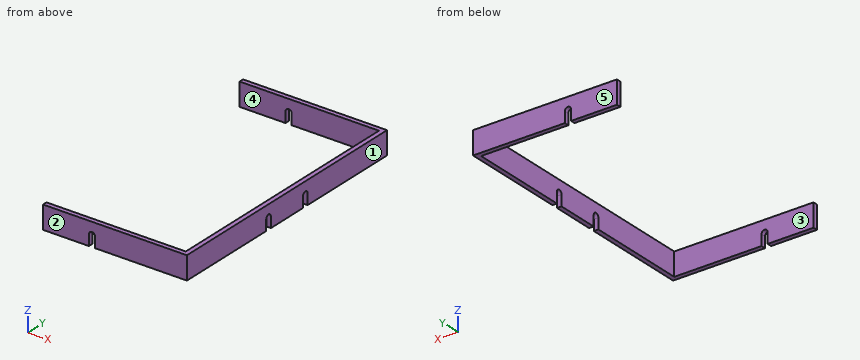
```python
from build123d import *

# Parameters (mm, degrees)
F0_W     = 94
F0_H     = 174
F1_DEPTH = 15
F2_T     = -3
F4_DEPTH = 100
F6_DEPTH = 125


with BuildPart() as f1:
    # F0 (on Top) → F1 (new body)
    with BuildSketch(Plane.XY):
        Rectangle(F0_W, F0_H)
    extrude(amount=F1_DEPTH)

    # F2
    f2_openings = [f1.faces().sort_by_distance(p)[0] for p in [
        (0, 0, 15),
        (-47, 0, 7.5),
        (0, 0, 0),
    ]]
    offset(amount=F2_T, openings=f2_openings)

    # F3 (on Right) → F4 (cut)
    with BuildSketch(Plane.YZ):
        with BuildLine():
            Line((-18, 7), (-14, 7))
            ThreePointArc((-14, 7), (-16, 9), (-18, 7))
        make_face()
        with BuildLine():
            Line((-14, 0), (-14, 7))
            ThreePointArc((-14, 7), (-16, 5), (-18, 7))
            Line((-18, 7), (-18, 0))
            Line((-18, 0), (-14, 0))
        make_face()
        with BuildLine():
            ThreePointArc((-18, 7), (-16, 5), (-14, 7))
            Line((-14, 7), (-18, 7))
        make_face()
        with BuildLine():
            Line((14, 7), (18, 7))
            ThreePointArc((18, 7), (16, 9), (14, 7))
        make_face()
        with BuildLine():
            Line((18, 0), (18, 7))
            ThreePointArc((18, 7), (16, 5), (14, 7))
            Line((14, 7), (14, 0))
            Line((14, 0), (18, 0))
        make_face()
        with BuildLine():
            ThreePointArc((14, 7), (16, 5), (18, 7))
            Line((18, 7), (14, 7))
        make_face()
    extrude(amount=F4_DEPTH, mode=Mode.SUBTRACT)

    # F5 (on Front) → F6 (cut, symmetric)
    with BuildSketch(Plane.XZ):
        with BuildLine():
            Line((-17, 7), (-13, 7))
            ThreePointArc((-13, 7), (-15, 9), (-17, 7))
        make_face()
        with BuildLine():
            Line((-13, 0), (-13, 7))
            ThreePointArc((-13, 7), (-15, 5), (-17, 7))
            Line((-17, 7), (-17, 0))
            Line((-17, 0), (-13, 0))
        make_face()
        with BuildLine():
            ThreePointArc((-17, 7), (-15, 5), (-13, 7))
            Line((-13, 7), (-17, 7))
        make_face()
    extrude(amount=F6_DEPTH, both=True, mode=Mode.SUBTRACT)


solid = f1.part
```
Geometry check sheet. Reference: the model listing, model coordinates, mm. Face numbers are marked on the shaded views. A direction names the side the tool comes from. Coordinates: 2 decimals unless noted, no trailing zeros. Write each loop counter-clockwise with the first axis right and the second up, starting at its lowest first coordinate (ties: lowest second). Pieces come first, ordered by that corner, then holes. Notation, with made-up numbers: M -32.75,-15 L 21.25,-15 A18 cw 21.25,-7 Z; hole C 3.25,55 d8. An arc over 180 degrees is marked long. Answer as a JSON object with one key per item and string values.
1. Draft check along Y on the marked faces 1, 2 and 3. Enter one of: released by +Y, released by -Y, zero draft, split by the parting line, or undercut.
Answers below:
{"face 1": "zero draft", "face 2": "released by -Y", "face 3": "undercut"}
2. Tool access check on the marked faces 4 and 5. Record the directions out of +Z, -Z, +X, -X, +Y, -Y that give a thin tool (end or side, any length) a straight path to the whole face; none if there is none.
Answers below:
{"face 4": "+Z, -Z, -X", "face 5": "+Z, -Z, +X, -X, +Y"}
3. Section check D-D, the plane y = -16. Enter the section's corners in (x, z), plus the area to 3 significant figures.
Answers below:
{"outline": "M 44,9 L 47,9 L 47,15 L 44,15 Z", "area": "18.0 mm²"}
4. Section check C-C, the plane x = -15. Enter the section's corners in (y, z).
Answers below:
{"outline": "M -87,9 L -84,9 L -84,15 L -87,15 Z; M 84,9 L 87,9 L 87,15 L 84,15 Z"}
5. Scan lines: L1, parallel to Y at x = 24.5, z = 7.25; L2, parallel to X at y = -76, z = 4. Record each from-to range of solid material in increasing order.
Answers below:
{"L1": "y = -87 to -84, 84 to 87", "L2": "x = 44 to 47"}
6. Go/stop test with a flat-tipped pin: pin 1 Ø4.5 at (y, z) = (-40.5, 4.5) entering from -X. Record where the tip stops, or that it passes through.
Answers below:
{"pin 1": "stops at x = 44"}
7. Section check A-A, the plane x = -2.5. Enter the section's corners in (y, z).
Answers below:
{"outline": "M -87,0 L -84,0 L -84,15 L -87,15 Z; M 84,0 L 87,0 L 87,15 L 84,15 Z"}
8. Section check B-B, the plane z = 2. Enter the section's corners in (x, y).
Answers below:
{"outline": "M -47,-87 L -17,-87 L -17,-84 L -47,-84 Z; M -47,84 L -17,84 L -17,87 L -47,87 Z; M -13,-87 L 47,-87 L 47,-18 L 44,-18 L 44,-84 L -13,-84 Z; M -13,84 L 44,84 L 44,18 L 47,18 L 47,87 L -13,87 Z; M 44,-14 L 47,-14 L 47,14 L 44,14 Z"}
